Part model, mm, in its own coordinate system. Round coordinates to 2 decimals unless told otherwise and drop trailing zeros. Loops run counter-clockwise (first coordinate to the right, second up) from the corner with the lowest first, then second, coordinate; pieces in that order, holes last. Notation, with made-up numbers: M 50.5,9 L 90.5,9 A18 ccw 90.5,27 Z; hole C 7,-12 d3. An arc over 180 degrees is marked long. Answer as CSV lines item,"result". Start each with the question number.
Item 1: Drop flat-ended pins along their axis: pin 1 Ø12 at (x, z) = (-52, -451.5) entering from -Y; pin 2 Ø1.5 at (y, z) = (52.5, -429.5) entering from +X; pin 3 Ø2 at (y, z) = (63, -495.5) entering from -X. Give the stop position or say it passes through.
Item 2: Band-saw the part on B-B (y = 63). Give the cut face in (x, z).
Item 3: Band-saw the part on A-A (x = -45.5). Give the cut face in (y, z).
Item 4: Wall check: line 1 (Y direction, x = -60, z = -448); line 2 (Y direction, x = -46, z = -434); line 3 (X direction, y = 56, z = -450.5). Give the ranges that are in metal, low to high.
```python
from build123d import *

# Parameters (mm, degrees)
BOSS_EXTRUDE1_START     = -392
BOSS_EXTRUDE1_DEPTH     = 147
CUT_EXTRUDE1_DEPTH      = 148
SKETCH3_OUTSIDE_W       = 81.897
SKETCH3_OUTSIDE_H       = 179.984
CUT_EXTRUDE2_DEPTH      = 26.581353828
CUT_EXTRUDE2_DEPTH_BACK = 23.337511723


with BuildPart() as part:
    # Sketch1 → Boss-Extrude1 (new body)
    with BuildSketch(Plane.XY.offset(BOSS_EXTRUDE1_START)):
        with BuildLine():
            Line((0, 76), (0, 78.6))
            ThreePointArc((0, 78.6), (-78.6, 0), (0, -78.6))
            Line((0, -78.6), (0, -76))
            ThreePointArc((0, -76), (-76, 0), (0, 76))
        make_face()
    extrude(amount=-BOSS_EXTRUDE1_DEPTH)

    # Sketch2 → Cut-Extrude1 (cut, through all)
    with BuildSketch(Plane.XY.offset(-392)):
        with BuildLine():
            Line((0, 0), (-28.679315249, 73.180987127))
            ThreePointArc((-28.679315249, 73.180987127), (49.357896331, -61.169911474), (-65.46760952, 43.496575771))
            Line((-65.46760952, 43.496575771), (0, 0))
        make_face()
    extrude(amount=-CUT_EXTRUDE1_DEPTH, mode=Mode.SUBTRACT)

    # Sketch3 outside → Cut-Extrude2 (cut, two sides)
    with BuildSketch(Plane(origin=(-45.516324952, 56.408999874, 0), x_dir=(0.778243149, 0.627963058, 0), z_dir=(-0.627963058, 0.778243149, 0))) as cut_extrude2_sk:
        with Locations((-0.0825, 465.5)):
            Rectangle(SKETCH3_OUTSIDE_W, SKETCH3_OUTSIDE_H)
        Polygon((23.635475841, 392), (-97.818058366, 392), (-57.320280341, 551.13514832), (-9.635475841, 539), (23.635475841, 420), align=None, mode=Mode.SUBTRACT)
    extrude(amount=CUT_EXTRUDE2_DEPTH, mode=Mode.SUBTRACT)
    extrude(cut_extrude2_sk.sketch, amount=-CUT_EXTRUDE2_DEPTH_BACK, mode=Mode.SUBTRACT)


solid = part.part
```
Answer block:
1,pin 1,"stops at y = 49.11"
1,pin 2,"stops at x = -54.23"
1,pin 3,"stops at x = -48.31"
2,outline,"M -47,-493.86 L -42.51,-481.36 L -42.51,-392 L -47,-392 Z"
3,outline,"M 60.87,-494.46 L 64.09,-487.24 L 64.09,-392 L 60.87,-392 Z"
4,line 1,"y = 46.65 to 50.77"
4,line 2,"y = 60.5 to 63.73"
4,line 3,"x = -55.15 to -51.38"
